Geometry: see drawing. Coordinates: mm, zero at the bounding-box minimum. Coordinates: 2 decimals unless noted, no trailing zeros. Write each loop counter-clockwise with the first axis right and the second up, starting at its lowest first coordinate (ties: lowest second). Pieces come first, ordered by that corner, then holes. Notation, with made-up numbers: M 55.25,85.5 L 101.25,85.5 A25 ccw 101.25,98.5 Z; hole C 22.25,-26 d6. An arc over 180 degrees is marked long. Answer as CSV lines item,"result". Start each with the question number.
1. Contact query for flat-ended pins moving along their axis: pin 1 Ø2 at (x, y) = (42, 9.5) entering from -Z; pin 2 Ø10 at (y, z) = (74.5, 27) entering from +X; pin 3 Ø4 at (x, z) = (48, 45) entering from -Y; pin 4 Ø4.5 at (x, y) = (19, 19.5) entering from -Z. Output: stop coordinate, or through.
2. Line query: probe 1 along Y at (x, z) = (42.5, 4); probe 2 along X at (y, z) = (33.5, 43); probe 3 along X at (y, z) = (53, 22). Output: solid intervals per line, ascending. Write a range as [from, to].
3. Section D-D on y = 10. Return the cut outline in (x, z), plus the area to 3 significant figures.
4. Section A-A on y = 42.5. Return the cut outline in (x, z).
5. Section C-C on z = 39. Return the cut outline in (x, y).
6. Section B-B on x = 26. Return the cut outline in (y, z).
7. Mould query, pull axis Y, two halves, no side actions, for the marked faces 1, 2 and 3. Classes: pulls with the +Y half, pulls with the -Y half, needs draft (parallel to the pull), parting line crosses it, or undercut.
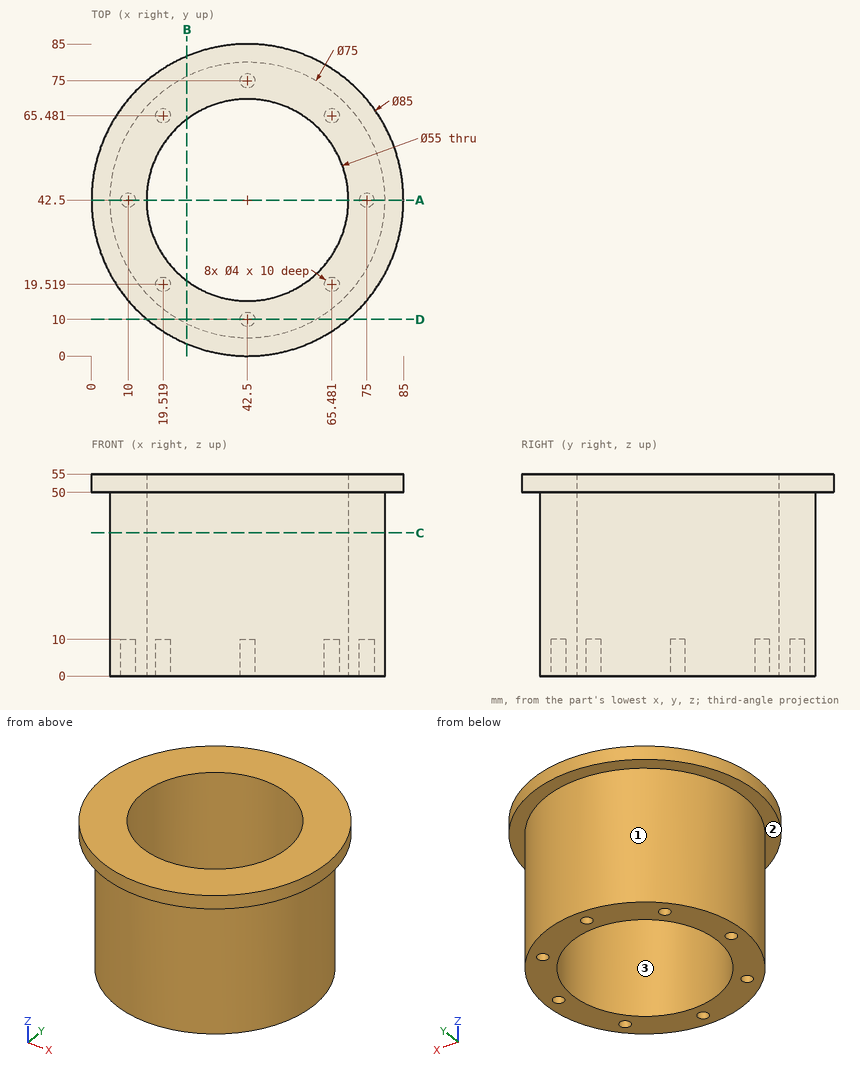
Values:
1,pin 1,"z = 10"
1,pin 2,"x = 68.52"
1,pin 3,"y = 5.16"
1,pin 4,"z = 0"
2,probe 1,"[5, 8], [12, 15], [70, 73], [77, 80]"
2,probe 2,"[6.1, 16.51], [68.49, 78.9]"
2,probe 3,"[6.5, 17.08], [67.92, 78.5]"
3,outline,"M 15.11,50 L 23.79,50 L 23.79,0 L 40.5,0 L 40.5,10 L 44.5,10 L 44.5,0 L 61.21,0 L 61.21,50 L 69.89,50 L 69.89,55 L 15.11,55 Z"
3,area,"2,100 mm²"
4,outline,"M 0,50 L 5,50 L 5,0 L 8,0 L 8,10 L 12,10 L 12,0 L 15,0 L 15,55 L 0,55 Z; M 70,0 L 73,0 L 73,10 L 77,10 L 77,0 L 80,0 L 80,50 L 85,50 L 85,55 L 70,55 Z"
5,outline,"C 42.5,42.5 d75; hole C 42.5,42.5 d55"
6,outline,"M 3.33,50 L 8.83,50 L 8.83,0 L 20.5,0 L 20.5,55 L 3.33,55 Z; M 64.5,0 L 76.17,0 L 76.17,50 L 81.67,50 L 81.67,55 L 64.5,55 Z"
7,face 1,"parting line crosses it"
7,face 2,"needs draft"
7,face 3,"undercut"
